from build123d import *

# Parameters (mm, degrees)
SKETCH1_W           = 60
SKETCH1_H           = 20
BOSS_EXTRUDE1_DEPTH = 12
SHELL1_T            = -1
SKETCH2_W           = 12.5
SKETCH2_H           = 4.7
CUT_EXTRUDE1_DEPTH  = 12
SKETCH3_W           = 19.267308131
SKETCH3_H           = 2.75
SKETCH3_R           = 0.75
SKETCH3_W_2         = 2.75
BOSS_EXTRUDE2_DEPTH = 4.5
FILLET1_R           = 5
FILLET2_R           = 5


with BuildPart() as part:
    # Sketch1 → Boss-Extrude1 (new body)
    with BuildSketch(Plane(origin=(0, 0, 0), x_dir=(1, 0, 0), z_dir=(0, 1, 0))):
        Rectangle(SKETCH1_W, SKETCH1_H)
    extrude(amount=BOSS_EXTRUDE1_DEPTH)

    # Shell1
    shell1_openings = [part.faces().sort_by_distance(p)[0] for p in [
        (0, 12, 0),
    ]]
    offset(amount=SHELL1_T, openings=shell1_openings, kind=Kind.INTERSECTION)

    # Sketch2 → Cut-Extrude1 (cut)
    with BuildSketch(Plane(origin=(30, 0, 0), x_dir=(0, 0, -1), z_dir=(1, 0, 0))):
        with Locations((0, 3.35)):
            Rectangle(SKETCH2_W, SKETCH2_H)
    extrude(amount=-CUT_EXTRUDE1_DEPTH, mode=Mode.SUBTRACT)

    # Sketch3 → Boss-Extrude2 (add)
    # profile 1 of 4: a face of its own
    with BuildSketch(Plane(origin=(0, 1, 0), x_dir=(1, 0, 0), z_dir=(0, 1, 0))):
        with Locations((19.366345935, 7.625)):
            Rectangle(SKETCH3_W, SKETCH3_H)
        with Locations(Location((26.5, 7.625, 0), (0, 0, 270))):
            Circle(SKETCH3_R, mode=Mode.SUBTRACT)
    # profile 2 of 4: a face of its own
    with BuildSketch(Plane(origin=(0, 1, 0), x_dir=(1, 0, 0), z_dir=(0, 1, 0))):
        with Locations((-27.625, 7.625)):
            Rectangle(SKETCH3_W_2, SKETCH3_H)
        with Locations(Location((-27.625, 7.625, 0), (0, 0, 270))):
            Circle(SKETCH3_R, mode=Mode.SUBTRACT)
    # profile 3 of 4: a face of its own
    with BuildSketch(Plane(origin=(0, 1, 0), x_dir=(1, 0, 0), z_dir=(0, 1, 0))):
        with Locations((-27.625, -7.625)):
            Rectangle(SKETCH3_W_2, SKETCH3_H)
        with Locations(Location((-27.625, -7.625, 0), (0, 0, 90))):
            Circle(SKETCH3_R, mode=Mode.SUBTRACT)
    # profile 4 of 4: a face of its own
    with BuildSketch(Plane(origin=(0, 1, 0), x_dir=(1, 0, 0), z_dir=(0, 1, 0))):
        with Locations((19.366345935, -7.625)):
            Rectangle(SKETCH3_W, SKETCH3_H)
        with Locations(Location((26.5, -7.625, 0), (0, 0, 90))):
            Circle(SKETCH3_R, mode=Mode.SUBTRACT)
    extrude(amount=BOSS_EXTRUDE2_DEPTH)

    # Fillet1
    # the kernel refuses this fillet: 5 mm, written as the material it adds along each edge
    with BuildSketch(Plane(origin=(-26.25, 1, 9), x_dir=(1, 0, 0), z_dir=(0, 0, -1))) as fillet1_piece_1:
        with BuildLine():
            CenterArc((4.974937186, -5), FILLET1_R, 90, 84.260829523)
            Line((0, -4.5), (-0.099498744, -4.49))
            ThreePointArc((-0.099498744, -4.49), (-0.1, -2.25), (-0.1, 0))
            Line((-0.1, 0), (0, 0.1))
            Line((0, 0.1), (4.974937186, 0.1))
            Line((4.974937186, 0.1), (4.974937186, 0))
        make_face()
    extrude(amount=2.75)
    with BuildSketch(Plane(origin=(-26.25, 1, -9), x_dir=(1, 0, 0), z_dir=(0, 0, 1)), Plane(origin=(9.732691869, 1, 9), x_dir=(-1, 0, 0), z_dir=(0, 0, -1))) as fillet1_piece_2:
        with BuildLine():
            CenterArc((4.974937186, 5), FILLET1_R, 185.739170477, 84.260829523)
            Line((0, 4.5), (-0.099498744, 4.49))
            ThreePointArc((-0.099498744, 4.49), (-0.1, 2.25), (-0.1, 0))
            Line((-0.1, 0), (0, -0.1))
            Line((0, -0.1), (4.974937186, -0.1))
            Line((4.974937186, -0.1), (4.974937186, 0))
        make_face()
    extrude(amount=2.75)
    with BuildSketch(Plane(origin=(9.732691869, 1, -9), x_dir=(0, 1, 0), z_dir=(0, 0, 1))) as fillet1_piece_3:
        with BuildLine():
            CenterArc((5, 4.974937186), FILLET1_R, 180, 84.260829523)
            Line((0, 4.974937186), (-0.1, 4.974937186))
            Line((-0.1, 4.974937186), (-0.1, 0))
            Line((-0.1, 0), (0, -0.1))
            ThreePointArc((0, -0.1), (2.25, -0.1), (4.49, -0.099498744))
            Line((4.49, -0.099498744), (4.5, 0))
        make_face()
    extrude(amount=2.75)

    # Fillet2
    fillet2_edges = [part.edges().sort_by_distance(p)[0] for p in [
        (9.732691869, 5.5, -7.625),
        (9.732691869, 5.5, 7.625),
    ]]
    fillet(fillet2_edges, radius=FILLET2_R)


solid = part.part
Could you check a few things on this model? Use its own coordinates, in mm. A direction names the side the tool comes from. Give positions to 0.01 mm unless a question says otherwise; leave off trailing zeros. Order: outer loops, then holes, each group sorted by start corner. A loop starts at its lowest first (then second) coordinate and runs counter-clockwise, first axis right, second up. Notation, with made-up numbers: (-8.5, 37.5) - (17.5, 37.5) arc R9 cw to (17.5, 47.5) - close; hole circle Ø5 at (-36.75, 1.25). An arc over 180 degrees is marked (long way). Return JSON: item names as keys, results as strings. Group by question number.
Q1. Thinking about a two-plate mould opening in X: for faces 4 (the face through (26.5, 1, 7.6)), 5 (the face through (-27, 3, -6.25)), 6 (the face through (27.23, 3.22, 7.79)), which applies, pulls with the +X half, pulls with the -X half, needs draft (parallel to the pull), parting line crosses it, or undercut?
Q2. Suppose I cut it at A-A, the plane z = -4. Please give me the cut outline in (x, y).
Q3. Suppose I cut it at C-C, the plane x = 26.5. Please give me the cut outline in (y, z) (3 decimals).
Q4. Please list where these lines run through material, in increasing order: line 1 along X through (y, z) = (9, 6.75); line 2 along Z through (x, y) = (19, 8); line 3 along Y through (x, z) = (-13, 0.25). Write a range as [from, to].
Q5. Suppose I cut it at B-B, the plane y = 6.75. Please give me the cut outline in (x, z).
Q6. Will this pin go through, and if not, where does the flat tip stop? pin 1 Ø1.6 at (x, z) = (-27.5, -7.5) entering from +Y.
Q7. Suppose I cut it at D-D, the plane x = 0. Please give me the cut outline in (y, z).
Q8. Which directions (+Z, -Z, +X, -X, +Y, -Y) give clear straight access to the entire face, cutting with the end or side of a thin tool? Please do faces 1 (the face through (-27, 3, 6.25)), 2 (the face through (29.5, 5.7, 0.1)), 3 (the face through (26.5, 1, -7.6)).
Resolved:
{
 "1": {"face 4": "undercut", "face 5": "needs draft", "face 6": "undercut"},
 "2": {"outline": "(-30, 0) - (30, 0) - (30, 1) - (-29, 1) - (-29, 12) - (-30, 12) - close; (29, 5.7) - (30, 5.7) - (30, 12) - (29, 12) - close"},
 "3": {"outline": "(0, -10) - (12, -10) - (12, -9) - (5.5, -9) - (5.5, -8.375) - (1, -8.375) - (1, -6.875) - (5.5, -6.875) - (5.5, -6.25) - (1, -6.25) - (1, 6.25) - (5.5, 6.25) - (5.5, 6.875) - (1, 6.875) - (1, 8.375) - (5.5, 8.375) - (5.5, 9) - (12, 9) - (12, 10) - (0, 10) - close"},
 "4": {"line 1": "x = [-30, -29], [29, 30]", "line 2": "z = [-10, -9], [9, 10]", "line 3": "y = [0, 1]"},
 "5": {"outline": "(-30, -10) - (30, -10) - (30, 10) - (-30, 10) - close; hole (-29, -9) - (29, -9) - (29, 9) - (-29, 9) - close"},
 "6": {"pin 1": "stops at y = 5.5"},
 "7": {"outline": "(0, -10) - (12, -10) - (12, -9) - (1, -9) - (1, 9) - (12, 9) - (12, 10) - (0, 10) - close"},
 "8": {"face 1": "+X, +Y", "face 2": "+X", "face 3": "+Y"}
}
